```python
from build123d import *


with BuildPart() as f1:
    # F0 (on Front) → F1 (revolve)
    with BuildSketch(Plane.XZ):
        Polygon((0, 3.175), (0, 0), (50.8, 0), (50.8, 3.175), (47.240072, 3.175), align=None)
        with BuildLine():
            Line((47.240072, 3.175), (50.8, 3.175))
            ThreePointArc((50.8, 3.175), (52.31077, 21.393685), (41.581185, 36.195))
            Line((41.581185, 36.195), (39.666256, 33.655))
            ThreePointArc((39.666256, 33.655), (49.421995, 19.898164), (47.240072, 3.175))
        make_face()
        Polygon((39.666256, 33.655), (41.581185, 36.195), (33.413851, 36.195), (33.413851, 33.655), align=None)
    revolve(axis=Axis((0, 0, 4.551888), (0, 0, -1)))


solid = f1.part
```
Check sheet for the modelled part. Datum: model origin and axes. Units: mm. A direction names the side the tool comes from. Coordinates: 2 decimals unless noted, no trailing zeros. Write each loop counter-clockwise with the first axis right and the second up, starting at its lowest first coordinate (ties: lowest second). Pieces come first, ordered by that corner, then holes. Notation, with made-up numbers: (20, -9.5) -> (44, -9.5) arc R25 ccw to (44, 26.5) -> close; hole circle Ø6 at (38, 32). An arc over 180 degrees is marked (long way). Use a Markdown table: item, result.
1. Sectioned sample at D-D (z = 19). Enter the section's corners in (x, y).
Reported:
| item | result |
|---|---|
| outline | circle Ø105.72 at (0, 0); hole circle Ø99.25 at (0, 0) |
2. Go/stop test with flat-tipped pins: pin 1 Ø2 at (x, y) = (26, -11) entering from +Z (3 decimals); pin 2 Ø1.5 at (x, z) = (-9, 27) entering from -Y; pin 3 Ø4 at (x, z) = (-19, 12) entering from -Y. Record where each tip stops, or that it passes through.
Reported:
| item | result |
|---|---|
| pin 1 | stops at z = 3.175 |
| pin 2 | stops at y = -49.63 |
| pin 3 | stops at y = -50.41 |
3. Scan lines: line 1 along Z through (x, y) = (-3.5, 35.5) (3 decimals); line 2 along Z through (x, y) = (6, 9) (3 decimals); line 3 along X through (y, z) = (-18.5, 21). Record each from-to range of solid material in increasing order.
Reported:
| item | result |
|---|---|
| line 1 | z = 0 to 3.175, 33.655 to 36.195 |
| line 2 | z = 0 to 3.175 |
| line 3 | x = -49.04 to -45.5, 45.5 to 49.04 |
4. Tool access check on faces 1 (the cylindrical face through (-7.24, 32.62, 34.91)), 2 (the flat face through (18, 29, 33.655)), 3 (the flat face through (0, -34, 36.195)). Record the directions out of +Z, -Z, +X, -X, +Y, -Y that give a thin tool (end or side, any length) a straight path to the whole face; none if there is none.
Reported:
| item | result |
|---|---|
| face 1 | +Z |
| face 2 | none |
| face 3 | +Z, +X, -X, +Y, -Y |
5. Release check for a two-part mould opening along X. For faces 4 (the cylindrical face through (-11.012, 49.592, 1.61)), 5 (the flat face through (1, -1, 0)), 6 (the flat face through (-1, -1, 3.175)) record: pulls with the +X half, pulls with the -X half, needs draft (parallel to the pull), parting line crosses it, or undercut.
Reported:
| item | result |
|---|---|
| face 4 | parting line crosses it |
| face 5 | needs draft |
| face 6 | undercut |
6. Sectioned sample at A-A (x = 0). Enter the section's corners in (y, z) (3 decimals), plus the area to 3 significant figures.
Reported:
| item | result |
|---|---|
| outline | (-50.8, 0) -> (50.8, 0) -> (50.8, 3.175) arc R26.298 ccw to (41.581, 36.195) -> (33.414, 36.195) -> (33.414, 33.655) -> (39.666, 33.655) arc R23.123 cw to (47.24, 3.175) -> (-47.24, 3.175) arc R23.123 cw to (-39.666, 33.655) -> (-33.414, 33.655) -> (-33.414, 36.195) -> (-41.581, 36.195) arc R26.298 ccw to (-50.8, 3.175) -> close |
| area | 587 mm2 |
7. Sectioned sample at C-C (z = 7). Enter the section's corners in (x, y), plus the area to 3 significant figures.
Reported:
| item | result |
|---|---|
| outline | circle Ø104.48 at (0, 0); hole circle Ø97.83 at (0, 0) |
| area | 1,060 mm2 |
